```python
from build123d import *

# Parameters (mm, degrees)
F0_R     = 2.6
F1_DEPTH = 10
F2_W     = 30
F2_H     = 14
F3_DEPTH = 7
F4_W     = 8.5
F4_H     = 4.3
F5_DEPTH = 25
F6_R     = 2.6
F7_DEPTH = 4


with BuildPart() as f1:
    # F0 (on Top) → F1 (new body)
    with BuildSketch(Plane.XY):
        with BuildLine():
            ThreePointArc((27, 0), (24.949747, 4.949747), (20, 7))
            Line((20, 7), (-20, 7))
            ThreePointArc((-20, 7), (-24.949747, 4.949747), (-27, 0))
            ThreePointArc((-27, 0), (-24.949747, -4.949747), (-20, -7))
            Line((-20, -7), (20, -7))
            ThreePointArc((20, -7), (24.949747, -4.949747), (27, 0))
        make_face()
        with Locations((-20, 0)):
            Circle(F0_R, mode=Mode.SUBTRACT)
        with Locations((20, 0)):
            Circle(F0_R, mode=Mode.SUBTRACT)
    extrude(amount=F1_DEPTH)

    # F2 (on face) → F3 (cut)
    with BuildSketch(Plane.XY.offset(10)):
        Rectangle(F2_W, F2_H)
    extrude(amount=-F3_DEPTH, mode=Mode.SUBTRACT)

    # F4 (on face) → F5 (cut)
    with BuildSketch(Plane.XY.offset(3)):
        with Locations((-7.75, -1.85)):
            Rectangle(F4_W, F4_H)
        with Locations((7.75, -1.85)):
            Rectangle(F4_W, F4_H)
    extrude(amount=-F5_DEPTH, mode=Mode.SUBTRACT)

    # F6 (on face) → F7 (cut)
    with BuildSketch(Plane(origin=(0, 0, 0), x_dir=(1, 0, 0), z_dir=(0, 0, -1))):
        Polygon((-15.9, -2.367136), (-15.9, 2.367136), (-20, 4.734272), (-24.1, 2.367136), (-24.1, -2.367136), (-20, -4.734272), align=None)
        with Locations((-20, 0)):
            Circle(F6_R, mode=Mode.SUBTRACT)
        Polygon((15.9, 2.367136), (15.9, -2.367136), (20, -4.734272), (24.1, -2.367136), (24.1, 2.367136), (20, 4.734272), align=None)
        with Locations((20, 0)):
            Circle(F6_R, mode=Mode.SUBTRACT)
    extrude(amount=-F7_DEPTH, mode=Mode.SUBTRACT)


solid = f1.part
```
The model under review builds one solid part; all positions refer to its coordinate system, in mm. A direction names the side the tool comes from. Round coordinates to 2 decimals unless told otherwise and drop trailing zeros. Loops run counter-clockwise (first coordinate to the right, second up) from the corner with the lowest first, then second, coordinate; pieces in that order, holes last. Notation, with made-up numbers: (46.25, 26.5) - (54.25, 26.5) arc R26 ccw to (54.25, 63.5) - close; hole circle Ø2 at (11.5, 68.5). An arc over 180 degrees is marked (long way). Write each question's results on one line, items separated by ' | '. Start each with the question number.
Q1. Draft analysis for pull direction X (two halves, no side actions). For faces 4 (the flat face through (-22.02, -3.57, 1.97)), 5 (the flat face through (0, 0, 0)), state which applies: pulls with the +X half, pulls with the -X half, needs draft (parallel to the pull), parting line crosses it, or undercut.
Q2. Take a section at A-A on z = 4.5. Give the boundary of the cut face in (x, y).
Q3. Tool access review of faces 1 (the flat face through (0, 0, 3)), 2 (the flat face through (-17.921, -3.534, 1.972)), 3 (the flat face through (12, -2, 2)): name each direction out of +Z, -Z, +X, -X, +Y, -Y from which nothing blocks a thin tool from reaching the whole face with its end or side.
Q4. Take a section at D-D on y = -3.25. Give the boundary of the cut face in (x, z), plus the area to 3 significant figures.
Q5. Take a section at C-C on x = -11. Give the boundary of the cut face in (y, z).
Q6. Insertion check: P1, Ø3, axis at y = 5.5, z = 5.5, coming from the +X side; P2, Ø2, axis at x = -4.5, y = -5.5, coming from the +Z side; P3, Ø6, axis at y = -1, z = 5.5, coming from the +X side; P4, Ø3, axis at x = 20, y = 0, coming from the +Z side. Each pin has a flat end and moves straight along its axis. Give the tip position at first contact, or say it passes through.
Q7. Wall thickness on line 1 along X through (y, z) = (0.25, 7); line 2 along X through (y, z) = (-1.75, 8.75); line 3 along X through (y, z) = (2.5, 0.5): over which ranges is each line inside the solid? List them lowest first. Write a range as [from, to].
Q8. Take a section at B-B on y = -0.5. Give the number of separate pieces and of enclosed holes in the cut face, plus the area to 3 significant figures.
Data:
1) face 4: undercut | face 5: needs draft
2) outline: (-27, 0) arc R7 ccw to (-20, -7) - (-15, -7) - (-15, 7) - (-20, 7) arc R7 ccw to start; (15, -7) - (20, -7) arc R7 ccw to (27, 0) arc R7 ccw to (20, 7) - (15, 7) - close; hole circle Ø5.2 at (-20, 0); hole circle Ø5.2 at (20, 0)
3) face 1: +Z, +Y, -Y | face 2: -Z | face 3: +Z, -Z
4) outline: (-26.2, 0) - (-22.57, 0) - (-22.57, 4) - (-17.43, 4) - (-17.43, 0) - (-12, 0) - (-12, 3) - (-15, 3) - (-15, 10) - (-26.2, 10) - close; (-3.5, 0) - (3.5, 0) - (3.5, 3) - (-3.5, 3) - close; (12, 0) - (17.43, 0) - (17.43, 4) - (22.57, 4) - (22.57, 0) - (26.2, 0) - (26.2, 10) - (15, 10) - (15, 3) - (12, 3) - close | area: 222 mm²
5) outline: (-7, 0) - (-4, 0) - (-4, 3) - (-7, 3) - close; (0.3, 0) - (7, 0) - (7, 3) - (0.3, 3) - close
6) P1: stops at x = 25.74 | P2: stops at z = 3 | P3: stops at x = 27 | P4: passes through
7) line 1: x = [-27, -22.59], [-17.41, -15], [15, 17.41], [22.59, 27] | line 2: x = [-26.78, -21.92], [-18.08, -15], [15, 18.08], [21.92, 26.78] | line 3: x = [-26.54, -23.87], [-16.13, 16.13], [23.87, 26.54]
8) separate pieces: 5 | enclosed holes: 0 | area: 152 mm²
